from build123d import *

# Parameters (mm, degrees)
MODEL_R                 = 1.5
SALIENTE_EXTRUIR2_DEPTH = 3


with BuildPart() as part:
    # Model → Saliente-Extruir2 (new body)
    with BuildSketch(Plane.XY):
        Polygon((18.200296, 46.696699), (4.765267, 33.26167), (33.26167, 4.765267), (46.696699, 18.200296), (52, 12.896995), (52, 0), (0, 0), (0, 52), (12.896995, 52), align=None)
        with Locations((39.837763, 5.543084)):
            Circle(MODEL_R, mode=Mode.SUBTRACT)
        with Locations((46.625988, 12.33131)):
            Circle(MODEL_R, mode=Mode.SUBTRACT)
        with Locations((12.33131, 46.625988)):
            Circle(MODEL_R, mode=Mode.SUBTRACT)
        with Locations((5.543084, 39.837763)):
            Circle(MODEL_R, mode=Mode.SUBTRACT)
    extrude(amount=SALIENTE_EXTRUIR2_DEPTH)


solid = part.part
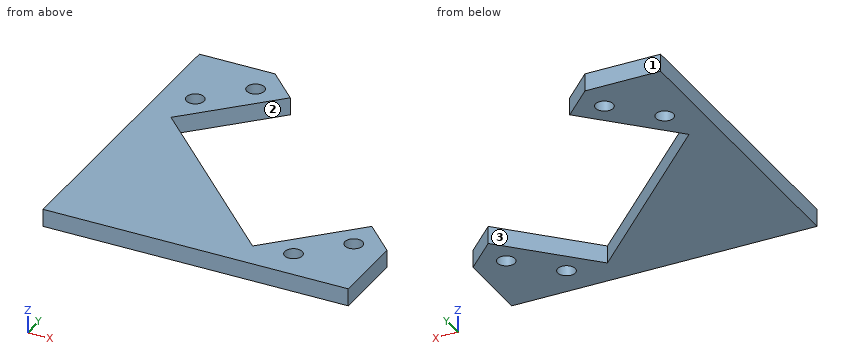
Verification items for the finished model (mm, model axes). Face numbers are marked on the shaded views. A direction names the side the tool comes from. Coordinates: 2 decimals unless noted, no trailing zeros. Order: outer loops, then holes, each group sorted by start corner. A loop starts at its lowest first (then second) coordinate and runs counter-clockwise, first axis right, second up. Notation, with made-up numbers: (31.25, -35.75) -> (90.25, -35.75) arc R31 cw to (90.25, 3.25) -> close; hole circle Ø5 at (0, 73). An arc over 180 degrees is marked (long way). Put each result on its own line as item: value. Start each with the question number.
1. Material ranges on L1, parallel to Y at x = 11.5, z = 1.1; L2, parallel to Y at x = 6.5, z = 1.7; L3, parallel to X at y = 11, z = 0.2, recorded low to high. Write a range as [from, to].
2. Cross-section at D-D, the plane x = 20.5. Record the boundary of the cut face in (y, z).
3. Go/stop test with a flat-tipped pin: pin 1 Ø12 at (x, y) = (20, 38) entering from -Z. Record where the tip stops, or that it passes through.
4. Cross-section at A-A, the plane x = 40.5. Record the boundary of the cut face in (y, z), then the cut area to 3 significant figures.
5. Access from +Z, -Z, +X, -X, +Y, -Y to the whole of each face (thin tool, end or side, straight path). Record for the marked faces 1, 2 and 3.
6. Cross-section at C-C, the plane z = 0.7. Record the boundary of the cut face in (x, y).
7. Cross-section at B-B, the plane y = 8. Record the boundary of the cut face in (x, z), then the cut area to 3 significant figures.
Computed:
1. L1: [0, 26.53], [40, 45.38], [47.87, 52]
1. L2: [0, 31.53], [35, 38.68], [40.99, 52]
1. L3: [0, 27.03], [39.5, 45.93], [47.32, 52]
2. outline: (0, 0) -> (17.53, 0) -> (17.53, 3) -> (0, 3) -> close
3. pin 1: through
4. outline: (0, 0) -> (4.2, 0) -> (4.2, 3) -> (0, 3) -> close; (6.89, 0) -> (12, 0) -> (12, 3) -> (6.89, 3) -> close
4. area: 27.9 mm2
5. face 1: +Z, -Z, +X, -X, +Y
5. face 2: +Z, -Z, +X
5. face 3: +Z, -Z, +Y
6. outline: (0, 0) -> (52, 0) -> (52, 12.9) -> (46.7, 18.2) -> (33.26, 4.77) -> (4.77, 33.26) -> (18.2, 46.7) -> (12.9, 52) -> (0, 52) -> close; hole circle Ø3 at (5.54, 39.84); hole circle Ø3 at (12.33, 46.63); hole circle Ø3 at (39.84, 5.54); hole circle Ø3 at (46.63, 12.33)
7. outline: (0, 0) -> (30.03, 0) -> (30.03, 3) -> (0, 3) -> close; (36.5, 0) -> (52, 0) -> (52, 3) -> (36.5, 3) -> close
7. area: 137 mm2
